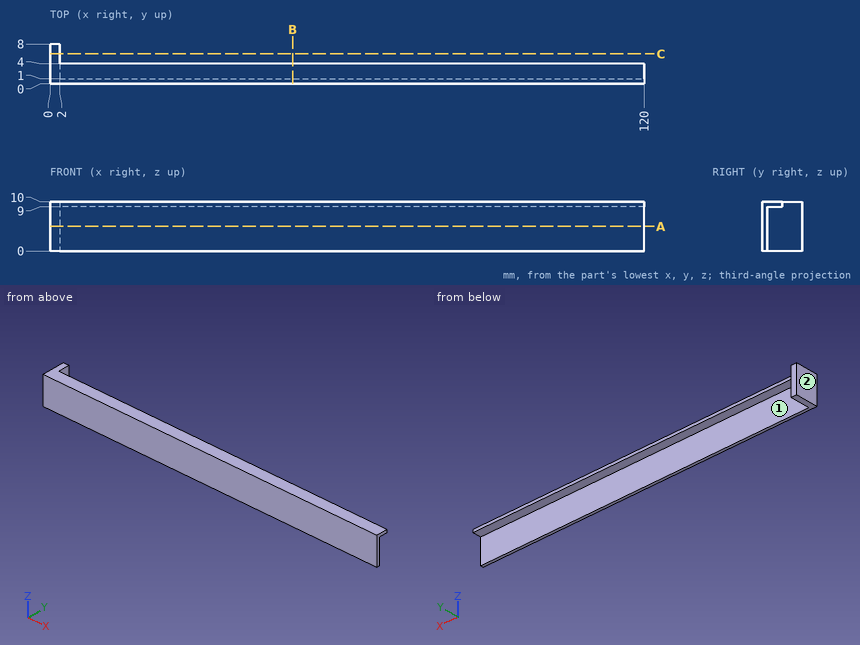
Study the drawing (mm; zero at the part's minimum x, y, z) and answer. A direction names the side the tool comes from. Give positions to 0.01 mm unless a question says otherwise; leave off trailing zeros. Loops run counter-clockwise (first coordinate to the right, second up) from the corner with the lowest first, then second, coordinate; pieces in that order, holes last. Notation, with made-up numbers: M 11,84.25 L 41,84.25 A19 ccw 41,102.25 Z; hole C 77,-20.75 d4. An arc over 180 degrees is marked long. Answer as CSV lines item,"result".
Item 1: The part is cut by section A-A (z = 5). Give the vertices of the cut face in (x, y).
Values follow:
outline,"M 0,0 L 120,0 L 120,1 L 2,1 L 2,8 L 0,8 Z"
Item 2: Which of the six approach directions +Z, -Z, +X, -X, +Y, -Y give full straight-line access (tool end or side, diameter ignored) to the marked faces 1 and 2?
Values follow:
face 1,"-Z, +X, +Y"
face 2,"+Z, -Z, -X, +Y, -Y"
Item 3: Straight lines are drawn through the part: line 1 along X through (y, z) = (4.75, 1); line 2 along Y through (x, z) = (29, 3); line 3 along Z through (x, y) = (108.5, 1.5). For each, find the intervals that lie inside material, in ascending order. Write a range as [from, to].
Values follow:
line 1,"x = [0, 2]"
line 2,"y = [0, 1]"
line 3,"z = [9, 10]"
Item 4: Given pin 1 Ø4.5 at (x, z) = (54.5, 3.5) entering from +Y; pin 2 Ø2 at (y, z) = (7, 5) entering from +X; pin 3 Ø3.5 at (x, y) = (50, 3) entering from -Z, each flat-ended and moving along its own axis, determine where each tip first touches the part or whether it passes through.
Values follow:
pin 1,"stops at y = 1"
pin 2,"stops at x = 2"
pin 3,"stops at z = 9"
Item 5: The part is cut by section B-B (x = 49). Give the vertices of the cut face in (y, z).
Values follow:
outline,"M 0,0 L 1,0 L 1,9 L 4,9 L 4,10 L 0,10 Z"
Item 6: The part is cut by section C-C (y = 6). Give the vertices of the cut face in (x, z).
Values follow:
outline,"M 0,0 L 2,0 L 2,10 L 0,10 Z"
